The model under review builds one solid part; all positions refer to its coordinate system, in mm. A direction names the side the tool comes from. Give positions to 0.01 mm unless a question says otherwise; leave off trailing zeros. Loops run counter-clockwise (first coordinate to the right, second up) from the corner with the lowest first, then second, coordinate; pieces in that order, holes last. Notation, with made-up numbers: M 50,23.25 L 72,23.25 A8 ccw 72,30.25 Z; hole C 88,-39 d2. An arc over 180 degrees is marked long. Return JSON: item names as keys, results as strings. Group by question number.
```python
from build123d import *

# Parameters (mm, degrees)
BASE_FLANGE1_START = -5
BASE_FLANGE1_DEPTH = 10
SKETCH6_R          = 2.5
CUT_EXTRUDE1_DEPTH = 10


# Read off the part's stored shape, not the designer's step: Base-Flange1
with BuildPart() as part:
    # Base-Flange1 outline → Base-Flange1 (new body)
    with BuildSketch(Plane.XY.offset(BASE_FLANGE1_START)):
        with BuildLine():
            Line((-16.314153364, 3), (-25, 3))
            Line((-25, 3), (-25, 0))
            Line((-25, 0), (-16.314153364, 0))
            ThreePointArc((-16.314153364, 0), (-13.985527754, 0.814326513), (-12.671868464, 2.902369657))
            ThreePointArc((-12.671868464, 2.902369657), (0, 13), (12.671868464, 2.902369657))
            ThreePointArc((12.671868464, 2.902369657), (13.985527754, 0.814326513), (16.314153364, 0))
            Line((16.314153364, 0), (25, 0))
            Line((25, 0), (25, 3))
            Line((25, 3), (16.314153364, 3))
            ThreePointArc((16.314153364, 3), (15.855108879, 3.160529066), (15.596145802, 3.57214727))
            ThreePointArc((15.596145802, 3.57214727), (0, 16), (-15.596145802, 3.57214727))
            ThreePointArc((-15.596145802, 3.57214727), (-15.855108879, 3.160529066), (-16.314153364, 3))
        make_face()
    extrude(amount=BASE_FLANGE1_DEPTH)

    # Sketch6 → Cut-Extrude1 (cut)
    with BuildSketch(Plane(origin=(0, 3, 0), x_dir=(1, 0, 0), z_dir=(0, 1, 0))):
        with Locations(Location((-20, 0, 0), (0, 0, 270))):
            Circle(SKETCH6_R)
    cut_extrude1 = extrude(amount=-CUT_EXTRUDE1_DEPTH, mode=Mode.SUBTRACT)

    # Mirror1: Cut-Extrude1 across plane
    add(cut_extrude1.mirror(Plane(origin=(0, 0, 0), x_dir=(0, 0, 1), z_dir=(1, 0, 0))), mode=Mode.SUBTRACT)


solid = part.part
```
(1) Add section A-A (z = 0). Write out the cut boundary in (x, y).
(2) Add section B-B (x = -20). Write out the cut boundary in (y, z), and give its area (3 significant figures).
(3) Mouldability with a two-part tool opening along Z and no side actions: class faces 4 (the cylindrical face through (0, 13, 0)), 5 (the flat face through (-0.1, 13.4, -5)), 6 (the cylindrical face through (17.52, 1.52, -0.33)) as released by +Z, released by -Z, zero draft, split by the parting line, or undercut.
(4) Add section C-C (y = 9). Write out the cut boundary in (x, z).
(5) For probe 1 along Z at (x, y) = (20, 1.65); probe 2 along X at (y, z) = (2.35, 0); probe 3 along X at (y, z) = (1.05, 0), list the stretches that pass through material, from the lowest coordinate up.
(6) For pin 1 (2.5 mm diameter, centred on x = 20, z = 1.5, fed in from +Y); pin 2 (2 mm diameter, centred on x = -16, z = 3, fed in from -Y); pin 3 (1.5 mm diameter, centred on y = 11, z = -4, fed in from +X); pin 4 (2 mm diameter, centred on x = -13, z = 4, fed in from -Y), all flat-tipped, find the tip position at first contact; note any pin that passes through.
(7) For faces 1 (the cylindrical face through (-14.013, 0.793, -0.07)), 2 (the flat face through (23, 3, 0)), 3 (the flat face through (-23, 3, 0)), list the 3-axis set-ups (+Z, -Z, +X, -X, +Y, -Y) from which the entire face can be reached by the end or side of a thin tool; tool diameter is ignored.
(8) Add section D-D (z = 3.75). Write out the cut boundary in (x, y).
Verdict:
{
 "1": {"outline": "M -25,0 L -22.5,0 L -22.5,3 L -25,3 Z; M -17.5,0 L -16.31,0 A3.74 ccw -12.67,2.9 A13 cw 12.67,2.9 A3.74 ccw 16.31,0 L 17.5,0 L 17.5,3 L 16.31,3 A0.74 cw 15.6,3.57 A16 ccw -15.6,3.57 A0.74 cw -16.31,3 L -17.5,3 Z; M 22.5,0 L 25,0 L 25,3 L 22.5,3 Z"},
 "2": {"outline": "M 0,-5 L 3,-5 L 3,-2.5 L 0,-2.5 Z; M 0,2.5 L 3,2.5 L 3,5 L 0,5 Z", "area": "15.0 mm²"},
 "3": {"face 4": "zero draft", "face 5": "released by -Z", "face 6": "undercut"},
 "4": {"outline": "M -13.23,-5 L -9.38,-5 L -9.38,5 L -13.23,5 Z; M 9.38,-5 L 13.23,-5 L 13.23,5 L 9.38,5 Z"},
 "5": {"probe 1": "z = -5 to -2.5, 2.5 to 5", "probe 2": "x = -25 to -22.5, -17.5 to -12.84, 12.84 to 17.5, 22.5 to 25", "probe 3": "x = -25 to -22.5, -17.5 to -13.72, 13.72 to 17.5, 22.5 to 25"},
 "6": {"pin 1": "stops at y = 3", "pin 2": "stops at y = 0", "pin 3": "stops at x = 12.29", "pin 4": "stops at y = 0.8"},
 "7": {"face 1": "+Z, -Z, -Y", "face 2": "+Z, -Z, +X, +Y", "face 3": "+Z, -Z, -X, +Y"},
 "8": {"outline": "M -25,0 L -16.31,0 A3.74 ccw -12.67,2.9 A13 cw 12.67,2.9 A3.74 ccw 16.31,0 L 25,0 L 25,3 L 16.31,3 A0.74 cw 15.6,3.57 A16 ccw -15.6,3.57 A0.74 cw -16.31,3 L -25,3 Z"}
}
